from build123d import *

# Parameters (mm, degrees)
SKIZZE1_W                       = 150
SKIZZE1_H                       = 175
AUFSATZ_LINEAR_AUSTRAGEN1_DEPTH = 10
SKIZZE2_R                       = 2.3876
SKIZZE2_R_2                     = 6.335
SCHNITT_LINEAR_AUSTRAGEN1_DEPTH = 10
SCHNITT_LINEAR_AUSTRAGEN2_DEPTH = 4
SKIZZE4_R                       = 1.25
SCHNITT_LINEAR_AUSTRAGEN3_DEPTH = 5
SCHNITT_LINEAR_START            = -5
SKIZZE6_R                       = 1.25
SCHNITT_LINEAR_AUSTRAGEN4_DEPTH = 5
SKIZZE7_R                       = 1
SCHNITT_LINEAR_AUSTRAGEN5_DEPTH = 40


with BuildPart() as part:
    # Skizze1 → Aufsatz-Linear austragen1 (new body)
    with BuildSketch(Plane.XY):
        with Locations((-21.140947697, -18.099765847)):
            Rectangle(SKIZZE1_W, SKIZZE1_H)
    extrude(amount=AUFSATZ_LINEAR_AUSTRAGEN1_DEPTH)

    # Skizze2 → Schnitt-Linear austragen1 (cut)
    with BuildSketch(Plane.XY.offset(10)):
        with Locations((-29.425704113, 26.900234153)):
            Circle(SKIZZE2_R)
        with Locations((-29.425704113, -63.099765847)):
            Circle(SKIZZE2_R_2)
    extrude(amount=-SCHNITT_LINEAR_AUSTRAGEN1_DEPTH, mode=Mode.SUBTRACT)

    # Skizze3 → Schnitt-Linear austragen2 (cut)
    with BuildSketch(Plane.XY.offset(10)):
        with BuildLine():
            Line((-54.425704113, 31.218234153), (-29.425704113, 31.218234153))
            ThreePointArc((-29.425704113, 31.218234153), (-26.372417032, 29.953521235), (-25.107704113, 26.900234153))
            Line((-25.107704113, 26.900234153), (-25.107704113, 1.900234153))
            ThreePointArc((-25.107704113, 1.900234153), (-23.842991195, -1.153052928), (-20.789704113, -2.417765847))
            Line((-20.789704113, -2.417765847), (8.756295887, -2.417765847))
            ThreePointArc((8.756295887, -2.417765847), (11.809582968, -1.153052928), (13.074295887, 1.900234153))
            Line((13.074295887, 1.900234153), (13.074295887, 69.400234153))
            Line((13.074295887, 69.400234153), (-58.743704113, 69.400234153))
            Line((-58.743704113, 69.400234153), (-58.743704113, 35.536234153))
            ThreePointArc((-58.743704113, 35.536234153), (-57.478991195, 32.482947072), (-54.425704113, 31.218234153))
        make_face()
    extrude(amount=-SCHNITT_LINEAR_AUSTRAGEN2_DEPTH, mode=Mode.SUBTRACT)

    # Skizze4 → Schnitt-Linear austragen3 (cut)
    with BuildSketch(Plane.ZY.offset(96.140947697)):
        with Locations(Location((5, 51.900234153, 0), (0, 0, 270))):
            Circle(SKIZZE4_R)
        with Locations(Location((5, -18.099765847, 0), (0, 0, 270))):
            Circle(SKIZZE4_R)
        with Locations(Location((5, -88.099765847, 0), (0, 0, 270))):
            Circle(SKIZZE4_R)
    extrude(amount=-SCHNITT_LINEAR_AUSTRAGEN3_DEPTH, mode=Mode.SUBTRACT)

    # Skizze6 → Schnitt-Linear austragen4 (cut)
    with BuildSketch(Plane(origin=(53.859052303, 0, 0), x_dir=(0, 0, -1), z_dir=(1, 0, 0)).offset(SCHNITT_LINEAR_START)):
        with Locations(Location((-5, 51.900234153, 0), (0, 0, 270))):
            Circle(SKIZZE6_R)
        with Locations(Location((-5, -18.099765847, 0), (0, 0, 270))):
            Circle(SKIZZE6_R)
        with Locations(Location((-5, -88.099765847, 0), (0, 0, 270))):
            Circle(SKIZZE6_R)
    extrude(amount=SCHNITT_LINEAR_AUSTRAGEN4_DEPTH, mode=Mode.SUBTRACT)

    # Skizze7 → Schnitt-Linear austragen5 (cut)
    with BuildSketch(Plane.XZ.offset(105.599765847)):
        with Locations(Location((-29.420947697, 5, 0), (0, 0, 270))):
            Circle(SKIZZE7_R)
    extrude(amount=-SCHNITT_LINEAR_AUSTRAGEN5_DEPTH, mode=Mode.SUBTRACT)


solid = part.part
CAD build for the part. Positions are in the model's coordinates, mm. A direction names the side the tool comes from. Give positions to 0.01 mm unless a question says otherwise; leave off trailing zeros. Write each loop counter-clockwise with the first axis right and the second up, starting at its lowest first coordinate (ties: lowest second). Pieces come first, ordered by that corner, then holes. Notation, with made-up numbers: M 63.5,24.25 L 121.5,24.25 A18 cw 121.5,51.25 Z; hole C 29.5,-30.5 d5. An arc over 180 degrees is marked long. Put each result on its own line as item: value. Start each with the question number.
(1) Probe L1, parallel to Y at x = 50.75, z = 5; L2, parallel to X at y = 7, z = 8.75; L3, parallel to X at y = -76.5, z = 5. List the from-to ranges inside material, lowest first.
(2) Mould opens along X. For faces 1 (the face through (-15, 42, 6)), 2 (the face through (-31.2, 28.5, 5.1)), 3 (the face through (-96.141, -19.3, 6)), 4 (the face through (-22, -36, 10)) say: +X half, -X half, draft (parallel to the pull), parting line (faces both ways), or undercut.
(3) Band-saw the part on A-A, the plane y = 42. Write the cut outline in (x, z).
(4) Band-saw the part on B-B, the plane x = -38.5. Write the cut outline in (y, z), and give its area (3 significant figures).
(5) Flat gauge pins, fed straight in: pin 1 Ø1.2 at (y, z) = (-88, 5.5) entering from -X; pin 2 Ø0.8 at (y, z) = (-18, 4.5) entering from +X. Where does each tip first touch, or does it go through?
(6) Band-saw the part on C-C, the plane y = 4.5. Write the cut outline in (x, z).
(7) Which spindle directions (+Z, -Z, +X, -X, +Y, -Y) get a long thin tool onto all of the face, cutting with end or side? Do faces 5 (the face through (-22, -17, 0)), 6 (the face through (-42, 31.218, 8)). Say none if no direction does.
Response values:
1. L1: y = -105.6 to -89.35, -86.85 to -19.35, -16.85 to 50.65, 53.15 to 69.4
1. L2: x = -96.14 to -25.11, 13.07 to 53.86
1. L3: x = -96.14 to -30.42, -28.42 to 53.86
2. face 1: undercut
2. face 2: undercut
2. face 3: -X half
2. face 4: draft
3. outline: M -96.14,0 L 53.86,0 L 53.86,10 L 13.07,10 L 13.07,6 L -58.74,6 L -58.74,10 L -96.14,10 Z
4. outline: M -105.6,0 L 69.4,0 L 69.4,6 L 31.22,6 L 31.22,10 L -105.6,10 Z
4. area: 1,600 mm2
5. pin 1: stops at x = -91.14
5. pin 2: stops at x = 48.86
6. outline: M -96.14,0 L 53.86,0 L 53.86,10 L 13.07,10 L 13.07,6 L -25.11,6 L -25.11,10 L -96.14,10 Z
7. face 5: -Z, +X, -X, +Y, -Y
7. face 6: +Z, +Y
